Autodesk Inventor part; units mm, degrees
ref_plane "YZ Plane" through (0, 0, 0) normal (1, 0, 0) x (0, 1, 0)
ref_plane "XZ Plane" through (0, 0, 0) normal (0, 1, 0) x (-1, 0, 0)
ref_plane "XY Plane" through (0, 0, 0) normal (0, 0, 1) x (1, 0, 0)
sketch "Náčrt1" plane through (0, 0, 0) normal (0, 0, 1) x (1, 0, 0)
  line L0 (-8, 0) -> (8, 0)
  line L1 (8, 0) -> (8, 27.5)
  line L2 (8, 27.5) -> (5.5, 27.5)
  line L3 (5.5, 27.5) -> (5.5, 26.5)
  line L4 (0.5, 21.5) -> (-0.5, 21.5)
  line L5 (-5.5, 26.5) -> (-5.5, 27.5)
  line L6 (-5.5, 27.5) -> (-8, 27.5)
  line L7 (-8, 27.5) -> (-8, 0)
  line L8 (-8, 16) -> (-6.3, 16)
  line L9 (-6.3, 16) -> (-6.3, 16.85)
  line L10 (-6.3, 16.85) -> (-5, 16.85)
  line L11 (-5, 16.85) -> (-5, 16)
  line L12 (-5, 16) -> (5, 16)
  line L13 (5, 16) -> (5, 14)
  line L14 (5, 14) -> (8, 14)
  arc A0 (-5.5, 26.5) -> (-0.5, 21.5) centre (-0.5, 26.5) ccw
  arc A1 (0.5, 21.5) -> (5.5, 26.5) centre (0.5, 26.5) ccw
  point P0 (0, 0)
  point P1 (0, 0)
  point P2 (5.5, 21.5)
  point P3 (-5.5, 21.5)
  dimension "d0" = 55
  dimension "d1" = 16
  dimension "d3" = 2.5
  dimension "d4" = 6
  dimension "d5" = 32
  dimension "d6" = 28
  dimension "d7" = 10
  dimension "d8" = 13
  dimension "d9" = 33.7
  dimension "d10" = 1.3
  dimension "d18" = 11
  dimension "d24" = 43
  dimension "d27" = 5
revolve "Rotace1" add sketch "Náčrt1" angle 360 about axis through (-8, 0, 0) along (1, 0, 0) contours L7 L6 L5 A0 L4 A1 L3 L2 L1 L14 L13 L12 L11 L10 L9 L8
chamfer "Zkosení1" distance 1 angle 45 1 edges at (-8, -16, 0)
chamfer "Zkosení2" distance 0.5 angle 45 5 edges at (-8, -27.5, 0) (-5.5, -27.5, 0) (5.5, -27.5, 0) (8, -27.5, 0) (8, -14, 0)
sketch "Náčrt2" plane through (8, 0, 0) normal (1, 0, 0) x (0, 0, -1)
  circle A0 centre (0, 0) radius 27.5
  circle A1 centre (0, 0) radius 14.5
  circle A2 centre (0, 0) radius 30
  dimension "d25" = 2.5
  dimension "d26" = 60
extrude "POLOTOVAR" [suppressed]
properties part number "DD_KVD_004_02" material "Nerezová ocel"
Build history of the part. All positions in model axes, mm. A direction names the side the tool comes from. Round coordinates to 2 decimals unless told otherwise and drop trailing zeros. Order: outer loops, then holes, each group sorted by start corner. A loop starts at its lowest first (then second) coordinate and runs counter-clockwise, first axis right, second up. Notation, with made-up numbers: (-19.75, 38) -> (1.25, 38) arc R28 ccw to (1.25, 61) -> close; hole circle Ø7 at (79, 38). An arc over 180 degrees is marked (long way). Answer in a Markdown table with one row per item.
1) Wall check: L1, parallel to X at y = 18, z = -20; L2, parallel to Z at x = -6.5, y = 0; L3, parallel to Z at x = 6.95, y = 0. Give the ranges that are in metal, low to high.
Values:
| item | result |
|---|---|
| L1 | -8 to -5.5, 5.5 to 8 |
| L2 | -27.5 to -16, 16 to 27.5 |
| L3 | -27.5 to -14, 14 to 27.5 |
2) Band-saw the part on A-A on x = -4.25. Give the cut face in (y, z), and give its area (3 significant figures).
Values:
| item | result |
|---|---|
| outline | circle Ø46.39 at (0, 0); hole circle Ø32 at (0, 0) |
| area | 886 mm2 |
3) Pin check, flat tips, straight feed: P1, Ø2, axis at x = -5, z = 20, coming from the +Y side; P2, Ø1.5, axis at x = 1.5, y = 18.5, coming from the +Z side; P3, Ø1.5, axis at x = 0.5, z = 15.5, coming from the -Y side; P4, Ø20, axis at y = 0, z = 0, coming from the +X side. Stop position of each tip, or through.
Values:
| item | result |
|---|---|
| P1 | y = 19.21 |
| P2 | z = 12.35 |
| P3 | y = -15.64 |
| P4 | through |
4) Band-saw the part on B-B on x = 3.25. Give the cut face in (y, z).
Values:
| item | result |
|---|---|
| outline | circle Ø44.65 at (0, 0); hole circle Ø32 at (0, 0) |
5) Mould opens along Y. For faces 4 (the flat face through (-8, 18, 0)), 5 (the flat face through (-5, 15, -6)), 6 (the cylindrical face through (-6.76, -5.961, 26.846)) say: released by +Y, released by -Y, zero draft, split by the parting line, or undercut.
Values:
| item | result |
|---|---|
| face 4 | zero draft |
| face 5 | undercut |
| face 6 | split by the parting line |
6) Which spindle directions (+Z, -Z, +X, -X, +Y, -Y) get a long thin tool onto all of the face, cutting with end or side? Do faces 1 (the flat face through (8, 12, -12)), 2 (the flat face through (-5.5, 17.9, -19.9)), 3 (the cylindrical face through (-6.65, -3.47, -15.62)). Say none if no direction does.
Values:
| item | result |
|---|---|
| face 1 | +Z, -Z, +X, +Y, -Y |
| face 2 | none |
| face 3 | -X |
